Part print with two shaded views. Sizes in mm from the minimum x, y, z corner. A direction names the side the tool comes from. Give positions to 0.01 mm unless a question says otherwise; leave off trailing zeros. Write each loop counter-clockwise with the first axis right and the second up, starting at its lowest first coordinate (ties: lowest second). Pieces come first, ordered by that corner, then holes. Notation, with made-up numbers: (60, 73.5) - (97, 73.5) arc R35 cw to (97, 109.5) - close; hole circle Ø11 at (-20, 73). An arc over 180 degrees is marked (long way). Answer as a JSON object with one key per item and string values. Group by question number.
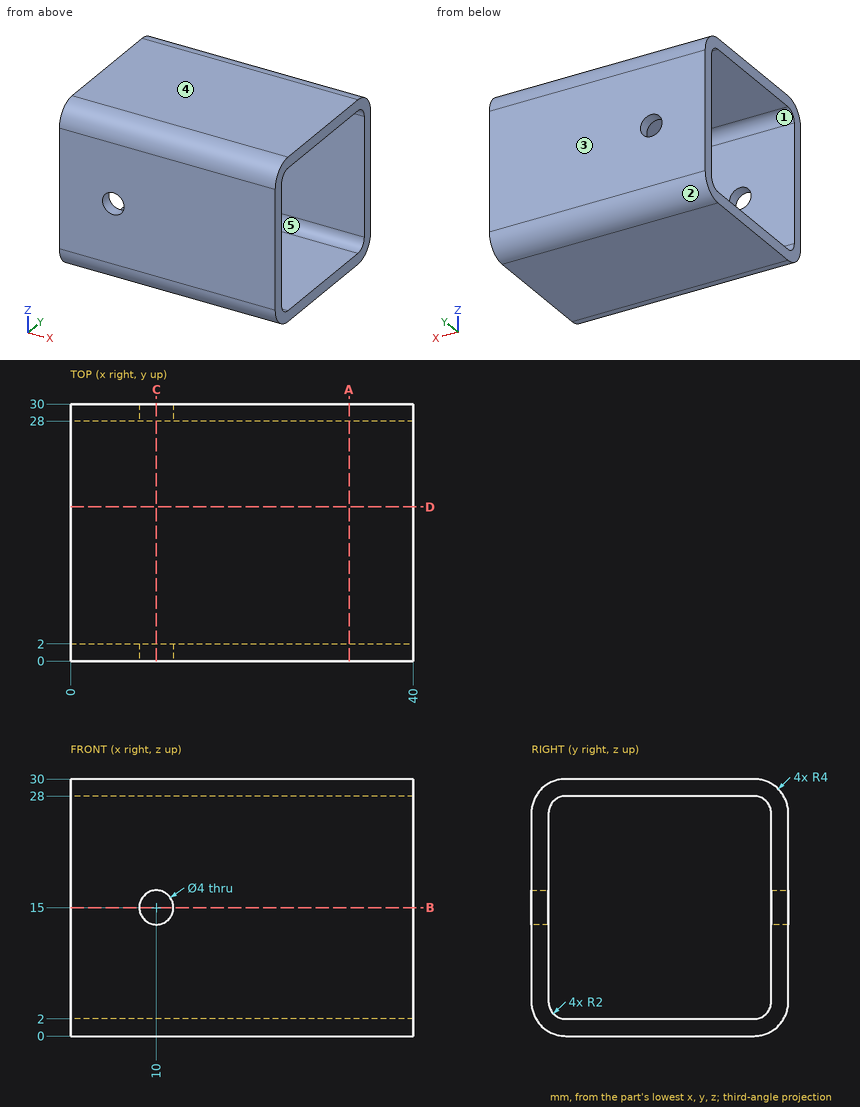
1) Which spindle directions (+Z, -Z, +X, -X, +Y, -Y) get a long thin tool onto all of the face, cutting with end or side? Do the marked faces 1 and 2. Say none if no direction does.
2) Drill centre lines: line 1 along Y through (x, z) = (10, 23.75); line 2 along X through (y, z) = (0.9, 15). Where is each one in solid material? Low to high. Write a range as from..to.
3) Two-plate mould, pull along Y, no slides. Class the marked faces 3, 4 and 5: +Y half, -Y half, draft (parallel to the pull), parting line (faces both ways), or undercut.
4) Saw through at D-D (y = 18). List the corners of the cut face in (x, z), and give its area (3 significant figures).
5) Saw through at A-A (x = 32.5). List the corners of the cut face in (y, z).
6) Saw through at B-B (z = 15). List the corners of the cut face in (x, y), and give its area (3 significant figures).
7) Saw through at C-C (x = 10). List the corners of the cut face in (y, z).
Checks:
{
 "1": {"face 1": "+X, -X", "face 2": "-Z, +X, -X, +Y"},
 "2": {"line 1": "0..2, 28..30", "line 2": "0..8, 12..40"},
 "3": {"face 3": "+Y half", "face 4": "draft", "face 5": "undercut"},
 "4": {"outline": "(0, 0) - (40, 0) - (40, 2) - (0, 2) - close; (0, 28) - (40, 28) - (40, 30) - (0, 30) - close", "area": "160 mm2"},
 "5": {"outline": "(0, 4) arc R4 ccw to (4, 0) - (26, 0) arc R4 ccw to (30, 4) - (30, 26) arc R4 ccw to (26, 30) - (4, 30) arc R4 ccw to (0, 26) - close; hole (2, 4) arc R2 ccw to (4, 2) - (26, 2) arc R2 ccw to (28, 4) - (28, 26) arc R2 ccw to (26, 28) - (4, 28) arc R2 ccw to (2, 26) - close"},
 "6": {"outline": "(0, 0) - (8, 0) - (8, 2) - (0, 2) - close; (0, 28) - (8, 28) - (8, 30) - (0, 30) - close; (12, 0) - (40, 0) - (40, 2) - (12, 2) - close; (12, 28) - (40, 28) - (40, 30) - (12, 30) - close", "area": "144 mm2"},
 "7": {"outline": "(0, 4) arc R4 ccw to (4, 0) - (26, 0) arc R4 ccw to (30, 4) - (30, 13) - (28, 13) - (28, 4) arc R2 cw to (26, 2) - (4, 2) arc R2 cw to (2, 4) - (2, 13) - (0, 13) - close; (0, 17) - (2, 17) - (2, 26) arc R2 cw to (4, 28) - (26, 28) arc R2 cw to (28, 26) - (28, 17) - (30, 17) - (30, 26) arc R4 ccw to (26, 30) - (4, 30) arc R4 ccw to (0, 26) - close"}
}
